from build123d import *

# Parameters (mm, degrees)
BOSS_EXTRUDE1_DEPTH          = 3
CUT_EXTRUDE1_DEPTH           = 133.140077191
CUT_EXTRUDE1_DEPTH_BACK      = 133.140077191
SKETCH2_R                    = 1.5
O_0_316_DIAMETER_HOLE1_D     = 8.0264
O_0_316_DIAMETER_HOLE1_DEPTH = 10
O_0_316_DIAMETER_HOLE1_TIP   = 2.411373836
SKETCH6_W                    = 140
SKETCH6_H                    = 10
CUT_EXTRUDE2_DEPTH           = 10
SKETCH7_R                    = 1.75
CUT_EXTRUDE3_DEPTH           = 10
BOSS_EXTRUDE3_DEPTH          = 6
FILLET2_R                    = 5


with BuildPart() as part:
    # Sketch1 → Boss-Extrude1 (new, symmetric)
    with BuildSketch(Plane.XY):
        with BuildLine():
            Line((-95, -60), (95, -60))
            ThreePointArc((95, -60), (102.071067812, -57.071067812), (105, -50))
            Line((105, -50), (105, 60))
            ThreePointArc((105, 60), (99.142135624, 74.142135624), (85, 80))
            Line((85, 80), (-85, 80))
            ThreePointArc((-85, 80), (-99.142135624, 74.142135624), (-105, 60))
            Line((-105, 60), (-105, -50))
            ThreePointArc((-105, -50), (-102.071067812, -57.071067812), (-95, -60))
        make_face()
        with BuildLine():
            Line((93, -1.00460734), (93, -38))
            ThreePointArc((93, -38), (90.071067812, -45.071067812), (83, -48))
            Line((83, -48), (20, -48))
            ThreePointArc((20, -48), (12.928932188, -45.071067812), (10, -38))
            Line((10, -38), (10, -35.031250653))
            ThreePointArc((10, -35.031250653), (10.691550782, -29.817443139), (12.71837888, -24.964196891))
            Line((12.71837888, -24.964196891), (32.056244976, 8.232176449))
            ThreePointArc((32.056244976, 8.232176449), (39.499751599, 14.924573129), (49.448622011, 16.026363354))
            Line((49.448622011, 16.026363354), (84.993679344, 8.794639706))
            ThreePointArc((84.993679344, 8.794639706), (90.743926441, 5.322445946), (93, -1.00460734))
        make_face(mode=Mode.SUBTRACT)
        with BuildLine():
            Line((-83, -48), (-20, -48))
            ThreePointArc((-20, -48), (-12.928932188, -45.071067812), (-10, -38))
            Line((-10, -38), (-10, -35.031250653))
            ThreePointArc((-10, -35.031250653), (-10.691550782, -29.817443139), (-12.71837888, -24.964196891))
            Line((-12.71837888, -24.964196891), (-32.056244976, 8.232176449))
            ThreePointArc((-32.056244976, 8.232176449), (-39.499751599, 14.924573129), (-49.448622011, 16.026363354))
            Line((-49.448622011, 16.026363354), (-84.993679344, 8.794639706))
            ThreePointArc((-84.993679344, 8.794639706), (-90.743926441, 5.322445946), (-93, -1.00460734))
            Line((-93, -1.00460734), (-93, -38))
            ThreePointArc((-93, -38), (-90.071067812, -45.071067812), (-83, -48))
        make_face(mode=Mode.SUBTRACT)
        with BuildLine():
            Line((-93, 31.650962878), (-93, 50))
            ThreePointArc((-93, 50), (-87.142135624, 64.142135624), (-73, 70))
            Line((-73, 70), (73, 70))
            ThreePointArc((73, 70), (87.142135624, 64.142135624), (93, 50))
            Line((93, 50), (93, 31.650962878))
            ThreePointArc((93, 31.650962878), (89.327053286, 23.907036437), (81.006320656, 21.851715832))
            Line((81.006320656, 21.851715832), (42.92968902, 29.598494092))
            ThreePointArc((42.92968902, 29.598494092), (40.946091564, 29.899370365), (38.942330332, 30))
            Line((38.942330332, 30), (-38.942330332, 30))
            ThreePointArc((-38.942330332, 30), (-40.946091564, 29.899370365), (-42.92968902, 29.598494092))
            Line((-42.92968902, 29.598494092), (-81.006320656, 21.851715832))
            ThreePointArc((-81.006320656, 21.851715832), (-89.327053286, 23.907036437), (-93, 31.650962878))
        make_face(mode=Mode.SUBTRACT)
    extrude(amount=BOSS_EXTRUDE1_DEPTH, both=True)

    # Sketch2 → Cut-Extrude1 (cut, two sides: drawn at the far end of the back side and taken through both)
    with BuildSketch(Plane.XY.offset(3).offset(-CUT_EXTRUDE1_DEPTH_BACK)):
        with Locations((100, 35)):
            Circle(SKETCH2_R)
        with Locations((100, -30)):
            Circle(SKETCH2_R)
        with Locations(Location((-100, -30, 0), (0, 0, 180))):
            Circle(SKETCH2_R)
        with Locations(Location((-100, 35, 0), (0, 0, 180))):
            Circle(SKETCH2_R)
    extrude(amount=CUT_EXTRUDE1_DEPTH + CUT_EXTRUDE1_DEPTH_BACK, mode=Mode.SUBTRACT)

    # O (0.316) Diameter Hole1
    with Locations(Plane.XY.offset(3)):
        with Locations((-19.247414599, 11.1125), (19.247414599, 11.1125), (0, -22.225)):
            Hole(O_0_316_DIAMETER_HOLE1_D / 2, depth=O_0_316_DIAMETER_HOLE1_DEPTH)
            with Locations((0, 0, -(O_0_316_DIAMETER_HOLE1_DEPTH + O_0_316_DIAMETER_HOLE1_TIP / 2))):  # 118° drill point
                Cone(0, O_0_316_DIAMETER_HOLE1_D / 2, O_0_316_DIAMETER_HOLE1_TIP, mode=Mode.SUBTRACT)

    # Sketch6 → Cut-Extrude2 (cut)
    with BuildSketch(Plane.XY.offset(3)):
        with Locations((0, 75)):
            Rectangle(SKETCH6_W, SKETCH6_H)
    extrude(amount=-CUT_EXTRUDE2_DEPTH, mode=Mode.SUBTRACT)

    # Sketch7 → Cut-Extrude3 (cut)
    with BuildSketch(Plane.XY.offset(3)):
        with Locations((-75, 75)):
            Circle(SKETCH7_R)
        with Locations((75, 75)):
            Circle(SKETCH7_R)
    extrude(amount=-CUT_EXTRUDE3_DEPTH, mode=Mode.SUBTRACT)

    # Sketch8 → Boss-Extrude3 (add)
    with BuildSketch(Plane(origin=(0, 0, -3), x_dir=(-1, 0, 0), z_dir=(0, 0, -1))):
        Polygon((-63.248850004, 80), (-70, 80), (-70, 70), (-25.96476149, 33.050047608), (-42.92968902, 29.598494092), (42.92968902, 29.598494092), (25.96476149, 33.050047608), (70, 70), (70, 80), (69.821528384, 80), (63.248850004, 80), (10.939239008, 36.107024707), (-10.939239008, 36.107024707), align=None)
    extrude(amount=-BOSS_EXTRUDE3_DEPTH)

    # Fillet2
    fillet2_edges = [part.edges().sort_by_distance(p)[0] for p in [
        (70, 70, 0),
        (-70, 70, 0),
        (25.96476149, 33.050047608, 0),
        (63.248850004, 80, 0),
        (10.939239008, 36.107024707, 0),
        (-10.939239008, 36.107024707, 0),
        (-63.248850004, 80, 0),
        (-25.96476149, 33.050047608, 0),
    ]]
    fillet(fillet2_edges, radius=FILLET2_R)


solid = part.part
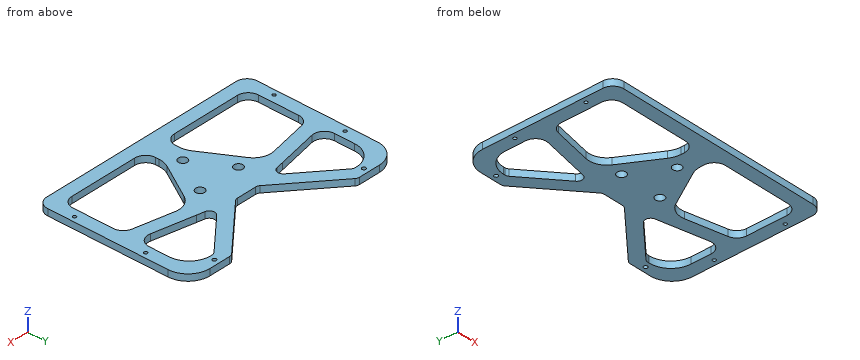
The model under review builds one solid part; all positions refer to its coordinate system, in mm. Round coordinates to 2 decimals unless told otherwise and drop trailing zeros. Write each loop counter-clockwise with the first axis right and the second up, starting at its lowest first coordinate (ties: lowest second). Pieces come first, ordered by that corner, then holes. Notation, with made-up numbers: (40, 36) -> (73, 36) arc R20 ccw to (73, 71) -> close; hole circle Ø2 at (41.25, 35). An arc over 180 degrees is marked (long way). Answer as a JSON object with one key per item and string values.
1. Clearance check with flat-ended pins moving along their axes: pin 1 (3 mm diameter, centred on x = 75, y = 75, fed in from -Z); pin 2 (13 mm diameter, centred on x = -19.25, y = 11.11, fed in from -Z); pin 3 (1.5 mm diameter, centred on x = 18, z = 1, fed in from +Y). State where each tip first meets the part, or that it passes through.
Results found:
{"pin 1": "passes through", "pin 2": "stops at z = -3", "pin 3": "stops at y = 42.66"}
2. We need section D-D on z = 0.1. State how many separate pieces and enclosed holes the cut face has, and give its area (3 significant figures).
Results found:
{"separate pieces": "1", "enclosed holes": "13", "area": "12,900 mm^2"}
3. We need section C-C on x = 51.5. State the section outline as (y, z) points, and give its area (3 significant figures).
Results found:
{"outline": "(-60, -3) -> (-48, -3) -> (-48, 3) -> (-60, 3) -> close; (15.61, -3) -> (27.85, -3) -> (27.85, 3) -> (15.61, 3) -> close; (54.48, -3) -> (70.14, -3) -> (70.14, 3) -> (54.48, 3) -> close", "area": "239 mm^2"}
4. We need section A-A on x = 0. State the section outline as (y, z) points.
Results found:
{"outline": "(-60, -3) -> (-26.24, -3) -> (-26.24, 3) -> (-60, 3) -> close; (-18.21, -3) -> (36.11, -3) -> (36.11, 3) -> (-18.21, 3) -> close"}
5. We need section B-B on y = 42. State the section outline as (x, z) points.
Results found:
{"outline": "(-105, -3) -> (-93, -3) -> (-93, 3) -> (-105, 3) -> close; (-36.63, -3) -> (-17.96, -3) -> (-17.96, 3) -> (-36.63, 3) -> close; (17.96, -3) -> (36.63, -3) -> (36.63, 3) -> (17.96, 3) -> close; (93, -3) -> (105, -3) -> (105, 3) -> (93, 3) -> close"}
6. To check wall thickness, follow line 1 along X through (y, z) = (-36.5, -0.2); line 2 along Y through (x, z) = (48.5, 0.55); line 3 along Y through (x, z) = (-100, -0.9). State the ranges of each line that lie inside material, in increasing order.
Results found:
{"line 1": "x = -105 to -93, -10 to 10, 93 to 105", "line 2": "y = -60 to -48, 16.19 to 28.47, 51.96 to 67.62", "line 3": "y = -58.66 to -31.5, -28.5 to 33.5, 36.5 to 73.23"}
